from build123d import *

# Parameters (mm, degrees)
F0_W     = 120
F0_H     = 80
F1_DEPTH = 40
F2_R     = 5
F4_DEPTH = 100


with BuildPart() as f1:
    # F0 (on Front) → F1 (new body)
    with BuildSketch(Plane.XZ):
        Rectangle(F0_W, F0_H)
    extrude(amount=F1_DEPTH)

    # F2
    f2_edges = [f1.edges().sort_by_distance(p)[0] for p in [
        (0, -40, 40),
        (0, -40, -40),
        (0, 0, 40),
        (0, 0, -40),
    ]]
    fillet(f2_edges, radius=F2_R)

    # F3 (on Right) → F4 (cut, symmetric)
    with BuildSketch(Plane.YZ):
        Polygon((-41.373981, 1.894575), (-38.208514, 1.82053), (-38.017184, 10), (-41.193411, 10), (-41.193411, 12), (-38.017184, 12), (-38.017184, 22), (-41.193411, 22), (-41.193411, 24), (-38.017184, 24), (-38.017184, 34), (-44.775072, 34), (-44.878796, 1.82053), (-44.878796, -1.82053), (-44.775072, -34), (-38.017184, -34), (-38.017184, -24), (-41.193411, -24), (-41.193411, -22), (-38.017184, -22), (-38.017184, -12), (-41.193411, -12), (-41.193411, -10), (-38.017184, -10), (-38.208514, -1.82053), (-41.373981, -1.823795), align=None)
    extrude(amount=F4_DEPTH, both=True, mode=Mode.SUBTRACT)


solid = f1.part
Input: part model. Units: mm. Frame: model coordinates. A direction names the side the tool comes from. Coordinates: 2 decimals unless noted, no trailing zeros. Loops run counter-clockwise (first coordinate to the right, second up) from the corner with the lowest first, then second, coordinate; pieces in that order, holes last. Notation, with made-up numbers: (72, -7) - (126, -7) arc R16 cw to (126, 16) - close; hole circle Ø5 at (24, -2.75). An arc over 180 degrees is marked (long way). Answer in a Markdown table with one row per item. Add a question column.
Item 1: Mould query, pull axis Z, two halves, no side actions, for faces 3 (the flat face through (1, -38.017, 17)), 4 (the cylindrical face through (1, -38, -39)), 5 (the flat face through (-1, -40, 0)). Classes: released by +Z, released by -Z, zero draft, split by the parting line, or undercut.
Item 2: Access query for faces 1 (the cylindrical face through (1, -2, 39)), 2 (the flat face through (1, -38.017, 29)). Directions: +Z, -Z, +X, -X, +Y, -Y. A direction counts if a zero-diameter tool reaches every point of the face in a straight line with its end or side. Return the directions, or none.
Item 3: Section query B-B on z = -19. Return the cut outline in (x, y), then the cut area to 3 significant figures.
Item 4: Contact query for flat-ended pins moving along their axis: P1, Ø5, axis at x = -18, z = -27.5, coming from the -Y side; P2, Ø0.6, axis at x = -8.5, y = -38.5, coming from the -Z side; P3, Ø1, axis at x = -27, y = -39.5, coming from the +Z side. Output: stop coordinate, or through.
Item 5: Line query: line 1 along Y through (x, z) = (-50, -26); line 2 along Y through (x, z) = (-32, -3); line 3 along Z through (x, y) = (-34, -3). Output: solid intervals per line, ascending. Write a range as [from, to].
Item 6: Section query C-C on z = 4. Return the cut outline in (x, y), then the cut area to 3 significant figures.
Recorded:
| question | item | result |
|---|---|---|
| 1 | face 3 | undercut |
| 1 | face 4 | released by -Z |
| 1 | face 5 | zero draft |
| 2 | face 1 | +Z, +X, -X, +Y |
| 2 | face 2 | +X, -X, -Y |
| 3 | outline | (-60, -38.02) - (60, -38.02) - (60, 0) - (-60, 0) - close |
| 3 | area | 4,560 mm^2 |
| 4 | P1 | y = -38.02 |
| 4 | P2 | z = -38.84 |
| 4 | P3 | z = 38 |
| 5 | line 1 | [-38.02, 0] |
| 5 | line 2 | [-38.18, 0] |
| 5 | line 3 | [-39.58, 39.58] |
| 6 | outline | (-60, -38.16) - (60, -38.16) - (60, 0) - (-60, 0) - close |
| 6 | area | 4,580 mm^2 |
